Check sheet for the drawn part. Datum: minimum x, y, z corner. Units: mm. Round coordinates to 2 decimals unless told otherwise and drop trailing zeros. Write each loop counter-clockwise with the first axis right and the second up, starting at its lowest first coordinate (ties: lowest second). Pieces come first, ordered by that corner, then holes. Notation, with made-up numbers: (56, 21.25) - (108, 21.25) arc R11 cw to (108, 25.25) - close; hole circle Ø10 at (3, -20.5). An arc over 180 degrees is marked (long way). Answer as a JSON object with one key per item and string values. Group by question number.
1) Section check B-B (y = 1.5). Enter the section's corners in (x, z), then the cut area to 3 significant figures.
2) Thickness scan on line 1 (Z direction, x = 32, y = 2.25); line 2 (Z direction, x = 584.2, y = 5.5); line 3 (X direction, y = 5.5, z = 31). Record the ranges inside material, lowest first.
3) Section check A-A (z = 19.05). Enter the section's corners in (x, y) (3 decimals).
4) Section check C-C (x = 584.2). Enter the section's corners in (y, z) (3 decimals).
5) Go/stop test with a flat-tipped pin: pin 1 Ø5 at (x, y) = (74.5, 6) entering from +Z. Record where the tip stops, or that it passes through.
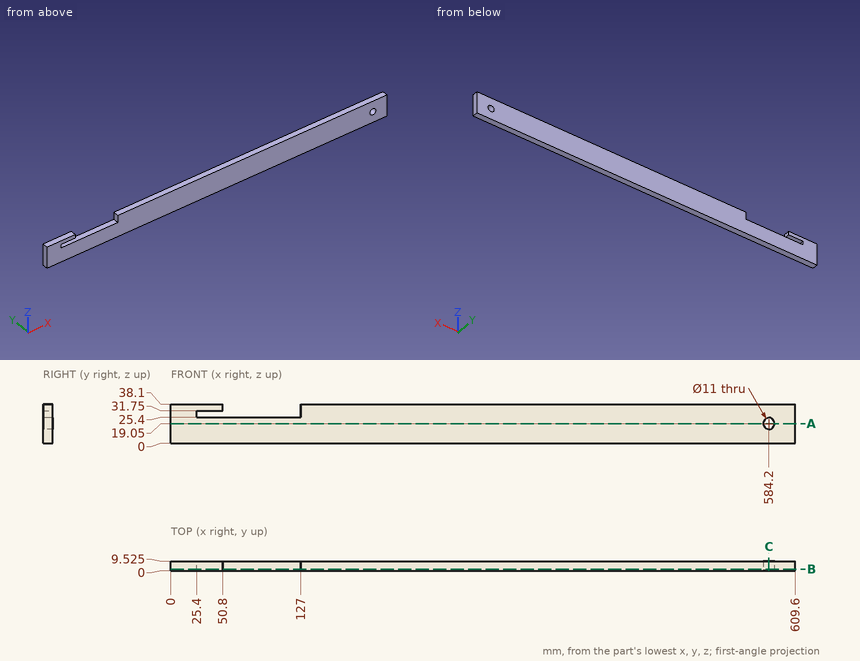
Returned:
{
 "1": {"outline": "(0, 0) - (609.6, 0) - (609.6, 38.1) - (127, 38.1) - (127, 25.4) - (25.4, 25.4) - (25.4, 31.75) - (50.8, 31.75) - (50.8, 38.1) - (0, 38.1) - close; hole circle Ø11 at (584.2, 19.05)", "area": "22,000 mm2"},
 "2": {"line 1": "0 to 25.4, 31.75 to 38.1", "line 2": "0 to 13.55, 24.55 to 38.1", "line 3": "0 to 25.4, 127 to 609.6"},
 "3": {"outline": "(0, 0) - (578.7, 0) - (578.7, 9.525) - (0, 9.525) - close; (589.7, 0) - (609.6, 0) - (609.6, 9.525) - (589.7, 9.525) - close"},
 "4": {"outline": "(0, 0) - (9.525, 0) - (9.525, 13.55) - (0, 13.55) - close; (0, 24.55) - (9.525, 24.55) - (9.525, 38.1) - (0, 38.1) - close"},
 "5": {"pin 1": "z = 25.4"}
}
